Study the drawing (mm; zero at the part's minimum x, y, z) and answer. Coordinates: 2 decimals unless noted, no trailing zeros. Loops run counter-clockwise (first coordinate to the right, second up) from the corner with the lowest first, then second, coordinate; pieces in that order, holes last. Notation, with made-up numbers: (80, 74) - (105, 74) arc R27 cw to (105, 111) - close; hole circle Ø7 at (16.25, 88.25). An arc over 180 degrees is marked (long way). Use CSV: the item, a comma, the result in double quotes.
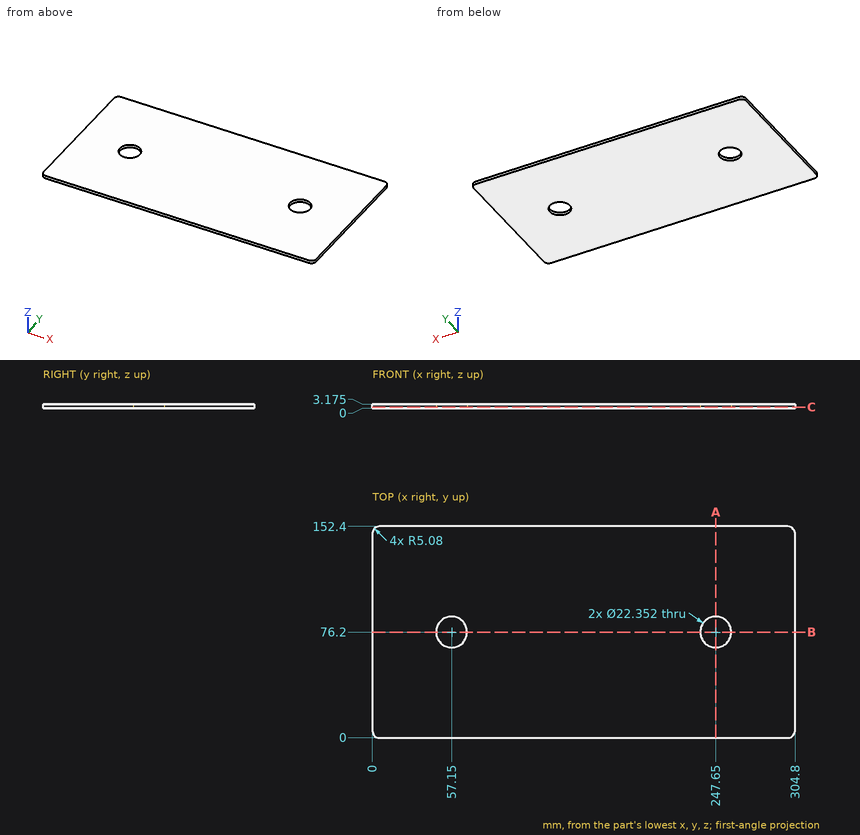
Q1. The part is cut by section C-C on z = 0.9. Determine the outline of the cut face in (x, y), and give its area (3 significant figures).
Reported:
outline,"(0, 5.08) arc R5.08 ccw to (5.08, 0) - (299.72, 0) arc R5.08 ccw to (304.8, 5.08) - (304.8, 147.32) arc R5.08 ccw to (299.72, 152.4) - (5.08, 152.4) arc R5.08 ccw to (0, 147.32) - close; hole circle Ø22.35 at (57.15, 76.2); hole circle Ø22.35 at (247.65, 76.2)"
area,"45,600 mm²"
Q2. The part is cut by section A-A on x = 247.65. Determine the outline of the cut face in (y, z) (3 decimals).
Reported:
outline,"(0, 0) - (65.024, 0) - (65.024, 3.175) - (0, 3.175) - close; (87.376, 0) - (152.4, 0) - (152.4, 3.175) - (87.376, 3.175) - close"
Q3. Find the intervals of material crossed by probe 1 along Y at (x, z) = (247.65, 2.2), in increasing order. Write a range as [from, to].
Reported:
probe 1,"y = [0, 65.02], [87.38, 152.4]"
Q4. Given P1, Ø13.5, axis at x = 247.65, y = 76.2, coming from the -Z side, flat-ended and moving along its own axis, determine where the tip first touches the part or whether it passes through.
Reported:
P1,"passes through"
Q5. The part is cut by section B-B on y = 76.2. Determine the outline of the cut face in (x, z) (3 decimals).
Reported:
outline,"(0, 0) - (45.974, 0) - (45.974, 3.175) - (0, 3.175) - close; (68.326, 0) - (236.474, 0) - (236.474, 3.175) - (68.326, 3.175) - close; (258.826, 0) - (304.8, 0) - (304.8, 3.175) - (258.826, 3.175) - close"
